Verification items for the finished model (mm, model axes). A direction names the side the tool comes from. Round coordinates to 2 decimals unless told otherwise and drop trailing zeros. Loops run counter-clockwise (first coordinate to the right, second up) from the corner with the lowest first, then second, coordinate; pieces in that order, holes last.
from build123d import *

# Parameters (mm, degrees)
F0_W     = 50
F0_H     = 50
F0_W_2   = 40
F0_H_2   = 40
F1_DEPTH = 35
F2_W     = 50
F2_H     = 50
F3_DEPTH = 25
F4_SIZE  = 24.99999
F5_W     = 40
F5_H     = 25
F6_DEPTH = 35
F8_W     = 49.4415648282
F8_H     = 49.9527305365
F9_DEPTH = 5


# Not quite as in the source:
# - a fillet or chamfer is up to 0.001 mm smaller than in the source, because OpenCascade refuses the exact size


with BuildPart() as f1:
    # F0 (on Top) → F1 (new body)
    with BuildSketch(Plane.XY):
        with Locations((25, 25)):
            Rectangle(F0_W, F0_H)
        with Locations((25, 25)):
            Rectangle(F0_W_2, F0_H_2, mode=Mode.SUBTRACT)
    extrude(amount=F1_DEPTH)

    # F2 (on face) → F3 (join)
    with BuildSketch(Plane.XY.offset(35)):
        with Locations((25, 25)):
            Rectangle(F2_W, F2_H)
    extrude(amount=F3_DEPTH)

    # F4 (size 25 in the source; OpenCascade refuses exactly that, so slightly less here)
    f4_edges = [f1.edges().sort_by_distance(p)[0] for p in [
        (0, 25, 60),
        (50, 25, 60),
    ]]
    chamfer(f4_edges, length=F4_SIZE)

    # F5 (on face) → F6 (cut)
    with BuildSketch(Plane.XZ):
        with Locations((25, 17.5)):
            Rectangle(F5_W, F5_H)
    extrude(amount=-F6_DEPTH, mode=Mode.SUBTRACT)

    # F8 (on face) → F9 (join)
    with BuildSketch(Plane(origin=(0, 0, 0), x_dir=(1, 0, 0), z_dir=(0, 0, -1))):
        with Locations((24.7207824141, -24.9763652682)):
            Rectangle(F8_W, F8_H)
    extrude(amount=F9_DEPTH)


solid = f1.part
1. Section check A-A (z = 31). Enter the section's corners in (x, y).
2. Tool access check on faces 4 (the face through (50, 25, 17)), 5 (the face through (25, 25, 0)), 6 (the face through (49.442, 25, -2)), 7 (the face through (0, 25, 15)), 8 (the face through (25, 2, 5)). Record the directions out of +Z, -Z, +X, -X, +Y, -Y that give a thin tool (end or side, any length) a straight path to the whole face; none if there is none.
3. Scan lines: L1, parallel to X at y = 21.5, z = 3.5; L2, parallel to Z at x = 35, y = 39.5; L3, parallel to Z at x = 25, y = 29.5. Record each from-to range of solid material in increasing order.
4. Section check C-C (z = 6). Enter the section's corners in (x, y), then the cut area to 3 significant figures.
5. Section check D-D (x = 16). Enter the section's corners in (y, z), then the cut area to 3 significant figures.
6. Release check for a two-part mould opening along Z. For faces 1 (the face through (5, 22, 17)), 2 (the face through (37, 25, 48)), 3 (the face through (24, 49.953, -2)) record: released by +Z, released by -Z, zero draft, split by the parting line, or undercut.
7. Gauge pin test, flat ends, axial feed: P1, Ø5.5, axis at y = 17.5, z = -3, coming from the +X side; P2, Ø1.5, axis at x = 34, z = -1.5, coming from the +Y side; P3, Ø10.5, axis at x = 34, z = 18, coming from the -Y side. Record the tip position at first contact, or that the pin passes through.
Taken from the geometry:
1. outline: (0, 0) - (50, 0) - (50, 50) - (0, 50) - close; hole (5, 5) - (45, 5) - (45, 45) - (5, 45) - close
2. face 4: +Z, -Z, +X, +Y, -Y
2. face 5: none
2. face 6: -Z, +X, +Y, -Y
2. face 7: +Z, -Z, -X, +Y, -Y
2. face 8: -Y
3. L1: x = 0 to 5, 45 to 50
3. L2: z = -5 to 0, 35 to 50
3. L3: z = -5 to 0, 35 to 60
4. outline: (0, 0) - (5, 0) - (5, 45) - (45, 45) - (45, 0) - (50, 0) - (50, 50) - (0, 50) - close
4. area: 700 mm2
5. outline: (0, -5) - (49.95, -5) - (49.95, 0) - (50, 0) - (50, 51) - (0, 51) - (0, 30) - (5, 30) - (5, 35) - (45, 35) - (45, 0) - (5, 0) - (5, 5) - (0, 5) - close
5. area: 1,270 mm2
6. face 1: undercut
6. face 2: released by +Z
6. face 3: zero draft
7. P1: stops at x = 49.44
7. P2: stops at y = 49.95
7. P3: stops at y = 45
